Input: dimensioned drawing with shaded views. Units: mm. Origin: part minimum x, y, z. Coordinates: 2 decimals unless noted, no trailing zeros. Loops run counter-clockwise (first coordinate to the right, second up) from the corner with the lowest first, then second, coordinate; pieces in that order, holes last.
Item 1: Section B-B on y = 2. Return loops of the section in (x, z) (1 decimal), and give its area (3 significant figures).
Item 2: Pull-direction query (X, two-part tool) for the marked faces 1, 2, 3 and 4; classes: released by +X, released by -X, zero draft, split by the parting line, or undercut.
Item 3: Ray query, line 1 along X through (y, z) = (5, 11) (1 decimal); line 2 along X through (y, z) = (3.5, 7) (1 decimal); line 3 along Z through (x, y) = (84.5, 10.5) (1 decimal). Return the intervals inside material, ascending.
Item 4: Contact query for flat-ended pins moving along their axis: P1, Ø2, axis at y = 7, z = 35, coming from the -X side; P2, Ø3, axis at y = 11, z = 25, coming from the -X side; P3, Ø2, axis at y = 6, z = 35, coming from the +X side (1 decimal). Output: stop coordinate, or through.
Item 5: Section A-A on z = 9. Return loops of the section in (x, y) (1 decimal), and give its area (3 significant figures).
Item 6: Section D-D on z = 40. Return loops of the section in (x, y) (1 decimal).
Item 7: Section C-C on y = 8.75. Return loops of the section in (x, z) (1 decimal), and give its area (3 significant figures).
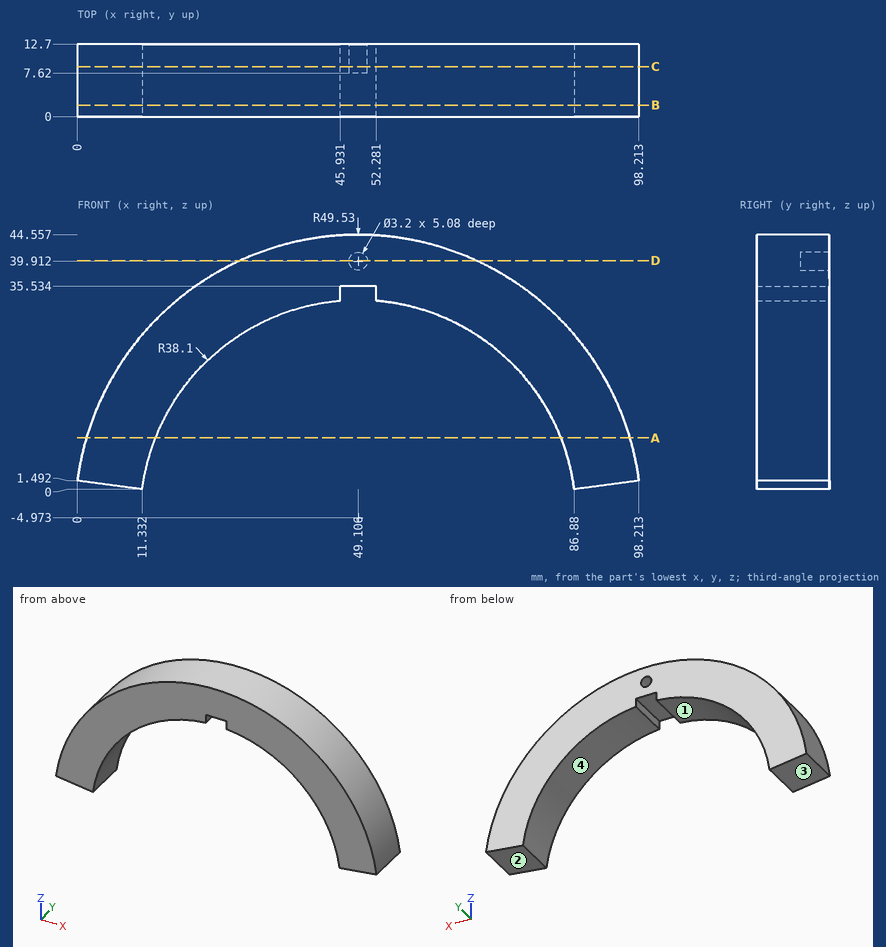
Results found:
1. outline: (0, 1.5) - (11.3, 0) arc R38.1 cw to (45.9, 33) - (45.9, 35.5) - (52.3, 35.5) - (52.3, 33) arc R38.1 cw to (86.9, 0) - (98.2, 1.5) arc R49.5 ccw to start
1. area: 1,430 mm2
2. face 1: undercut
2. face 2: released by +X
2. face 3: released by -X
2. face 4: undercut
3. line 1: x = 2.2 to 14.5, 83.7 to 96
3. line 2: x = 1 to 12.9, 85.3 to 97.2
3. line 3: z = 9.1 to 29.7
4. P1: stops at x = 18.54
4. P2: stops at x = 8.58
4. P3: stops at x = 79.7
5. outline: (1.6, 0) - (13.7, 0) - (13.7, 12.7) - (1.6, 12.7) - close; (84.6, 0) - (96.6, 0) - (96.6, 12.7) - (84.6, 12.7) - close
5. area: 307 mm2
6. outline: (28.4, 0) - (69.9, 0) - (69.9, 12.7) - (50.7, 12.7) - (50.7, 7.6) - (47.5, 7.6) - (47.5, 12.7) - (28.4, 12.7) - close
7. outline: (0, 1.5) - (11.3, 0) arc R38.1 cw to (45.9, 33) - (45.9, 35.5) - (52.3, 35.5) - (52.3, 33) arc R38.1 cw to (86.9, 0) - (98.2, 1.5) arc R49.5 ccw to start; hole circle Ø3.2 at (49.1, 39.9)
7. area: 1,420 mm2
